```python
from build123d import *

# Parameters (mm, degrees)
SKETCH_W        = 110
SKETCH_H        = 110
PAD_DEPTH       = 6
POCKET_DEPTH    = 110
POCKET001_DEPTH = 110


with BuildPart() as part:
    # Sketch → Pad (new body)
    with BuildSketch(Plane.XY):
        Rectangle(SKETCH_W, SKETCH_H)
    extrude(amount=PAD_DEPTH)

    # Sketch002 (on Face3 of Pad) → Pocket (cut)
    with BuildSketch(Plane.XZ.offset(55)):
        Polygon((55, 6), (55, 0), (49, 0), align=None)
        Polygon((-55, 6), (-55, 0), (-49, 0), align=None)
    extrude(amount=-POCKET_DEPTH, mode=Mode.SUBTRACT)

    # Sketch001 (on Face2 of Pad) → Pocket001 (cut)
    with BuildSketch(Plane.YZ.offset(55)):
        Polygon((-55, 6), (-55, 0), (-49, 0), align=None)
        Polygon((55, 6), (49, 0), (55, 0), align=None)
    extrude(amount=-POCKET001_DEPTH, mode=Mode.SUBTRACT)


solid = part.part
```
Design review of the part built by this model. Coordinates are the model's own, in mm. Round coordinates to 2 decimals unless told otherwise and drop trailing zeros. Order: outer loops, then holes, each group sorted by start corner. A loop starts at its lowest first (then second) coordinate and runs counter-clockwise, first axis right, second up. Notation, with made-up numbers: (-17, 21) - (1, 21) arc R15 cw to (1, 26) - close; hole circle Ø3 at (-0.5, 77.25). An arc over 180 degrees is marked (long way). Return JSON: item names as keys, results as strings.
Q1. For pin 1 Ø3 at (x, z) = (18.5, 2.5) entering from +Y; pin 2 Ø2 at (y, z) = (25.5, 1) entering from -X, all flat-tipped, find the tip position at first contact; note any pin that passes through.
Computed values:
{"pin 1": "stops at y = 53", "pin 2": "stops at x = -51"}
Q2. Wall thickness on L1, parallel to Y at x = -22, z = 4; L2, parallel to X at y = 46, z = 2; L3, parallel to X at y = 23, z = 4.75: over which ranges is each line inside the solid? List them lowest first. Write a range as [from, to].
Computed values:
{"L1": "y = [-53, 53]", "L2": "x = [-51, 51]", "L3": "x = [-53.75, 53.75]"}
Q3. Consider section A-A on y = -9.5. Write out the cut boundary in (x, z).
Computed values:
{"outline": "(-55, 6) - (-49, 0) - (49, 0) - (55, 6) - close"}
Q4. The part is to be moulded in two halves that separate along Z. For faces 1 (the flat face through (-1, 1, 6)), 2 (the flat face through (52, -1, 3)), say which applies: pulls with the +Z half, pulls with the -Z half, needs draft (parallel to the pull), parting line crosses it, or undercut.
Computed values:
{"face 1": "pulls with the +Z half", "face 2": "pulls with the -Z half"}
Q5. Consider section B-B on z = 3.5. Write out the cut boundary in (x, y).
Computed values:
{"outline": "(-52.5, -52.5) - (52.5, -52.5) - (52.5, 52.5) - (-52.5, 52.5) - close"}
